Design review of the part built by this model. Coordinates are the model's own, in mm. Face numbers are marked on the shaded views. A direction names the side the tool comes from. Give positions to 0.01 mm unless a question says otherwise; leave off trailing zeros. Write each loop counter-clockwise with the first axis right and the second up, starting at its lowest first coordinate (ties: lowest second). Pieces come first, ordered by that corner, then holes.
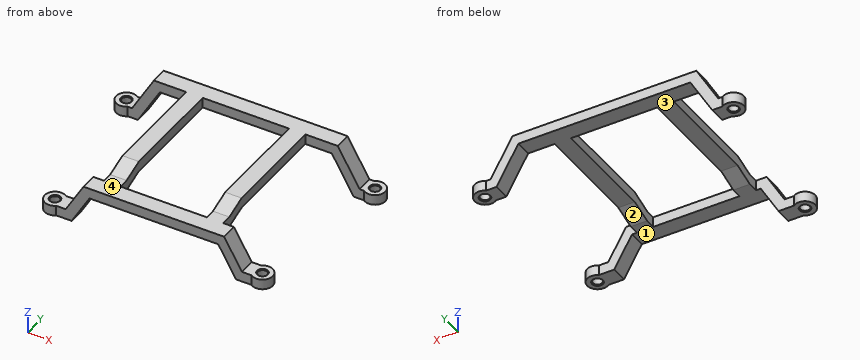
Solid Edge part; units mm, degrees
sketch "Sketch1" plane through (0, 0, 0) normal (0, 0, 1) x (1, 0, 0)
  circle A0 centre (-60.5, 0) radius 5
  circle A1 centre (60.5, 0) radius 5
  circle A2 centre (50.5, -75) radius 5
  circle A3 centre (-50.5, -75) radius 5
extrude "Protrusion1" add sketch "Sketch1" along normal blind 5
sketch "Sketch2" plane through (0, 0, 0) normal (0, -1, 0) x (1, 0, 0)
  line L0 (-60.5, 0) -> (-52.5, 0)
  line L1 (-52.5, 0) -> (-41.8397, 18.4641)
  line L2 (-41.8397, 18.4641) -> (41.8397, 18.4641)
  line L3 (41.8397, 18.4641) -> (52.5, 0)
  line L4 (52.5, 0) -> (60.5, 0)
  line L5 (60.5, 5) -> (60.5, 0)
  line L6 (60.5, 5) -> (55.3868, 5)
  line L7 (55.3868, 5) -> (44.7265, 23.4641)
  line L8 (44.7265, 23.4641) -> (-44.7265, 23.4641)
  line L9 (-44.7265, 23.4641) -> (-55.3868, 5)
  line L10 (-55.3868, 5) -> (-60.5, 5)
  line L11 (-60.5, 5) -> (-60.5, 0)
extrude "larger_bow" add sketch "Sketch2" along normal mid plane 8
sketch "Sketch3" plane through (0, -75, 0) normal (0, -1, 0) x (1, 0, 0)
  line L0 (-50.5, 5) -> (-50.5, 0)
  line L1 (-50.5, 0) -> (-40, 0)
  line L2 (-40, 0) -> (-31.3397, 15)
  line L3 (-31.3397, 15) -> (31.3397, 15)
  line L4 (31.3397, 15) -> (40, 0)
  line L5 (40, 0) -> (50.5, 0)
  line L6 (50.5, 0) -> (50.5, 5)
  line L7 (50.5, 5) -> (42.8868, 5)
  line L8 (42.8868, 5) -> (34.2265, 20)
  line L9 (34.2265, 20) -> (-34.2265, 20)
  line L10 (-34.2265, 20) -> (-42.8868, 5)
  line L11 (-42.8868, 5) -> (-50.5, 5)
extrude "smaller_bow" add sketch "Sketch3" along normal mid plane 8
hole "Hole1" at (60.5, 0, 5) direction (0, 0, -1) diameter 4.5 end up to next start chamfer 0.4 start chamfer angle 45 end chamfer 0.4 end chamfer angle 45
hole "Hole2" at (50.5, -75, 5) direction (0, 0, -1) diameter 4.5 end up to next start chamfer 0.4 start chamfer angle 45 end chamfer 0.4 end chamfer angle 45
hole "Hole3" at (-50.5, -75, 5) direction (0, 0, -1) diameter 4.5 end up to next start chamfer 0.4 start chamfer angle 45 end chamfer 0.4 end chamfer angle 45
hole "Hole4" at (-60.5, 0, 5) direction (0, 0, -1) diameter 4.5 end up to next start chamfer 0.4 start chamfer angle 45 end chamfer 0.4 end chamfer angle 45
sketch "Sketch4" plane through (25, 0, 0) normal (1, 0, 0) x (0, 1, 0)
  line L0 (-71, 20) -> (-66, 20)
  line L1 (-66, 20) -> (-56, 23.4641)
  line L2 (-56, 23.4641) -> (-4, 23.4641)
  line L3 (-4, 23.4641) -> (-4, 18.4641)
  line L4 (-4, 18.4641) -> (-56, 18.4641)
  line L5 (-56, 18.4641) -> (-66, 15)
  line L6 (-66, 15) -> (-71, 15)
  line L7 (-71, 15) -> (-71, 20)
  dimension "D1" = 71
  dimension "D2" = 66
extrude "ExtrudedProtrusion_4" add sketch "Sketch4" along normal mid plane 8
mirror "Mirror1" about plane through (0, 0, 0) normal (1, 0, 0) of "ExtrudedProtrusion_4"
properties material "Polyethylene, low density"
(1) To check wall thickness, follow L1, parallel to Y at x = 50.5, z = 1.7; L2, parallel to Z at x = -19.5, y = 1; L3, parallel to Y at x = 37, z = 5.5. State the ranges of each line that lie inside material, in increasing order.
Resolved:
L1: y = -80 to -77.25, -72.75 to -70
L2: z = 18.46 to 23.46
L3: y = -79 to -71
(2) Consider section B-B, the plane y = -35. Give the boundary of the cut face in (x, z), then the cut area to 3 significant figures.
Resolved:
outline: (-29, 18.46) - (-21, 18.46) - (-21, 23.46) - (-29, 23.46) - close; (21, 18.46) - (29, 18.46) - (29, 23.46) - (21, 23.46) - close
area: 80.0 mm2
(3) Consider section C-C, the plane y = -75. Give the boundary of the cut face in (x, z).
Resolved:
outline: (-55.5, 0) - (-53.15, 0) - (-52.75, 0.4) - (-52.75, 4.6) - (-53.15, 5) - (-55.5, 5) - close; (-48.25, 0.4) - (-47.85, 0) - (-40, 0) - (-31.34, 15) - (31.34, 15) - (40, 0) - (47.85, 0) - (48.25, 0.4) - (48.25, 4.6) - (47.85, 5) - (42.89, 5) - (34.23, 20) - (-34.23, 20) - (-42.89, 5) - (-47.85, 5) - (-48.25, 4.6) - close; (52.75, 0.4) - (53.15, 0) - (55.5, 0) - (55.5, 5) - (53.15, 5) - (52.75, 4.6) - close
(4) Consider section D-D, the plane x = -9.5. Give the boundary of the cut face in (y, z).
Resolved:
outline: (-79, 15) - (-71, 15) - (-71, 20) - (-79, 20) - close; (-4, 18.46) - (4, 18.46) - (4, 23.46) - (-4, 23.46) - close
(5) Mouldability with a two-part tool opening along X and no side actions: class the marked faces 3 and 4 as pulls with the +X half, pulls with the -X half, needs draft (parallel to the pull), parting line crosses it, or undercut.
Resolved:
face 3: undercut
face 4: needs draft
(6) Clearance check with flat-ended pins moving along their axes: P1, Ø7, axis at x = 60.5, y = 0, coming from the +Z side; P2, Ø4, axis at y = -42, z = 19, coming from the +X side; P3, Ø4, axis at x = -13, y = -72, coming from the -Z side. State where each tip first meets the part, or that it passes through.
Resolved:
P1: stops at z = 5
P2: stops at x = 29
P3: stops at z = 15
(7) Tool access review of the marked faces 1 and 2: name each direction out of +Z, -Z, +X, -X, +Y, -Y from which nothing blocks a thin tool from reaching the whole face with its end or side.
Resolved:
face 1: -Z, +Y, -Y
face 2: -Z, +X, -X, +Y
(8) Consider section A-A, the plane x = 60.5. Give the boundary of the cut face in (y, z).
Resolved:
outline: (-5, 0) - (-2.65, 0) - (-2.25, 0.4) - (-2.25, 4.6) - (-2.65, 5) - (-5, 5) - close; (2.25, 0.4) - (2.65, 0) - (5, 0) - (5, 5) - (2.65, 5) - (2.25, 4.6) - close
